Check sheet for the drawn part. Datum: minimum x, y, z corner. Units: mm. A direction names the side the tool comes from. Round coordinates to 2 decimals unless told otherwise and drop trailing zeros. Loops run counter-clockwise (first coordinate to the right, second up) from the corner with the lowest first, then second, coordinate; pieces in that order, holes last. Notation, with made-up numbers: (-9.75, 22.5) -> (38.25, 22.5) arc R4 cw to (38.25, 26.5) -> close; hole circle Ø1 at (14.5, -19). An arc over 180 degrees is marked (long way). Return JSON: item names as keys, results as strings.
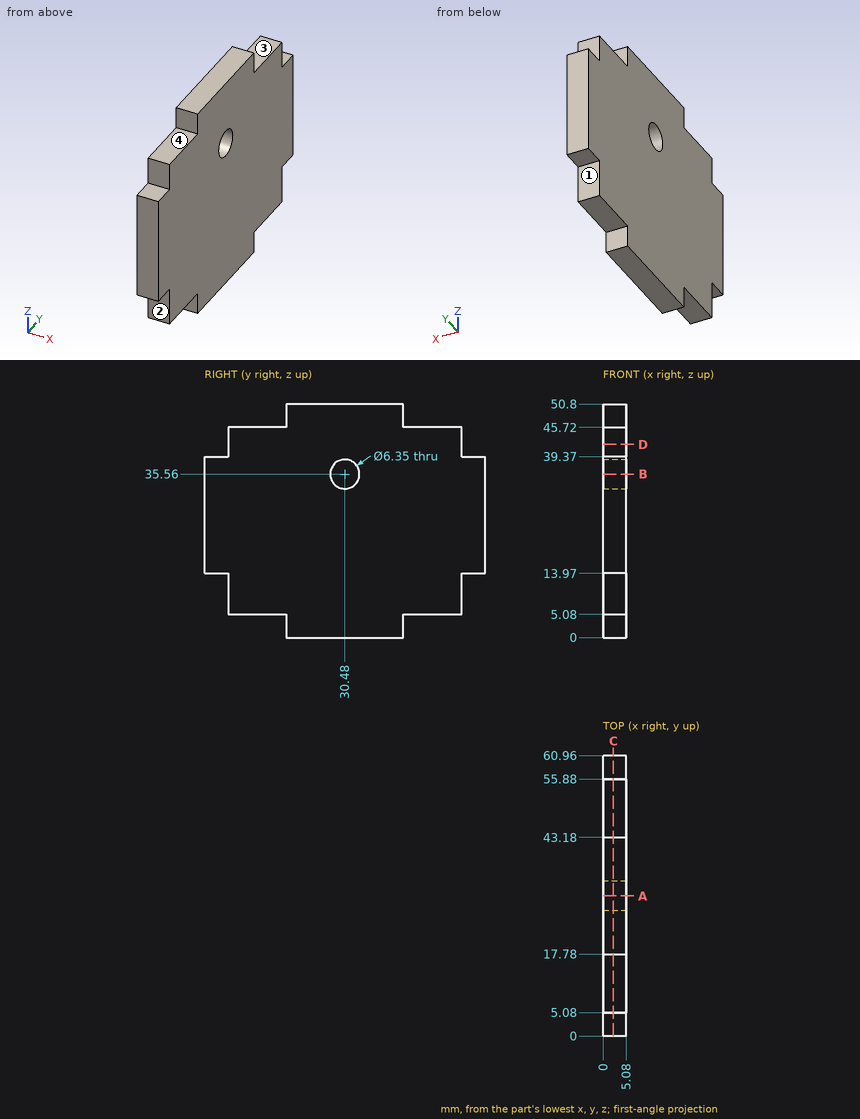
Q1. Material ranges on line 1 (Z direction, x = 1.9, y = 30.48) (3 decimals); line 2 (Z direction, x = 4.4, y = 12); line 3 (Y direction, x = 2.8, z = 5), recorded low to high.
Results list:
{"line 1": "0 to 32.385, 38.735 to 50.8", "line 2": "5.08 to 45.72", "line 3": "17.78 to 43.18"}
Q2. Go/stop test with flat-tipped pins: pin 1 (1.5 mm diameter, centred on x = 1.5, z = 11.5, fed in from -Y); pin 2 (1.5 mm diameter, centred on x = 2, y = 9, fed in from +Z); pin 3 (1.5 mm diameter, centred on x = 2, y = 47.5, fed in from -Z). Record where each tip stops, or that it passes through.
Results list:
{"pin 1": "y = 5.08", "pin 2": "z = 45.72", "pin 3": "z = 5.08"}
Q3. Section check C-C (x = 2.25). Record the boundary of the cut face in (y, z) (3 decimals), then the cut area to 3 significant figures.
Results list:
{"outline": "(0, 13.97) -> (5.08, 13.97) -> (5.08, 5.08) -> (17.78, 5.08) -> (17.78, 0) -> (43.18, 0) -> (43.18, 5.08) -> (55.88, 5.08) -> (55.88, 13.97) -> (60.96, 13.97) -> (60.96, 39.37) -> (55.88, 39.37) -> (55.88, 45.72) -> (43.18, 45.72) -> (43.18, 50.8) -> (17.78, 50.8) -> (17.78, 45.72) -> (5.08, 45.72) -> (5.08, 39.37) -> (0, 39.37) -> close; hole circle Ø6.35 at (30.48, 35.56)", "area": "2,550 mm^2"}
Q4. Section check B-B (z = 35.56). Record the boundary of the cut face in (x, y) (3 decimals), then the cut area to 3 significant figures.
Results list:
{"outline": "(0, 0) -> (5.08, 0) -> (5.08, 27.305) -> (0, 27.305) -> close; (0, 33.655) -> (5.08, 33.655) -> (5.08, 60.96) -> (0, 60.96) -> close", "area": "277 mm^2"}
Q5. Tool access check on the marked faces 1, 2, 3 and 4. Record the directions out of +Z, -Z, +X, -X, +Y, -Y that give a thin tool (end or side, any length) a straight path to the whole face; none if there is none.
Results list:
{"face 1": "-Z, +X, -X, +Y", "face 2": "-Z, +X, -X, -Y", "face 3": "+Z, +X, -X, +Y", "face 4": "+Z, +X, -X, -Y"}
Q6. Section check A-A (y = 30.48). Record the boundary of the cut face in (x, z) (3 decimals).
Results list:
{"outline": "(0, 0) -> (5.08, 0) -> (5.08, 32.385) -> (0, 32.385) -> close; (0, 38.735) -> (5.08, 38.735) -> (5.08, 50.8) -> (0, 50.8) -> close"}
Q7. Section check D-D (z = 42). Record the boundary of the cut face in (x, y), then the cut area to 3 significant figures.
Results list:
{"outline": "(0, 5.08) -> (5.08, 5.08) -> (5.08, 55.88) -> (0, 55.88) -> close", "area": "258 mm^2"}
